Work out the finished part from the listing and answer in its coordinate system (mm). A direction names the side the tool comes from. Coordinates: 2 decimals unless noted, no trailing zeros. Write each loop counter-clockwise with the first axis right and the second up, starting at its lowest first coordinate (ties: lowest second). Pieces come first, ordered by that corner, then holes. Notation, with made-up numbers: (15, 26) - (69, 26) arc R7 cw to (69, 36) - close; hole circle Ø3 at (57, 62.25). An arc over 180 degrees is marked (long way). Answer as a JSON object with one key per item and string values. Group by question number.
Autodesk Inventor part; units mm, degrees
ref_plane "YZ Plane" through (0, 0, 0) normal (1, 0, 0) x (0, 1, 0)
ref_plane "XZ Plane" through (0, 0, 0) normal (0, 1, 0) x (-1, 0, 0)
ref_plane "XY Plane" through (0, 0, 0) normal (0, 0, 1) x (1, 0, 0)
sketch "Sketch1" plane through (0, 0, 0) normal (1, 0, 0) x (0, 1, 0)
  line L0 (-10, 10) -> (10, 10)
  line L1 (10, 10) -> (10, -10)
  line L2 (10, -10) -> (-10, -10)
  line L3 (-10, -10) -> (-10, 10)
  line L4 (-10, 10) -> (10, -10) construction
  line L5 (10, 10) -> (-10, -10) construction
  line L6 (7, -7) -> (7, 7)
  line L7 (7, 7) -> (-7, 7)
  line L8 (-7, 7) -> (-7, -7)
  line L9 (-7, -7) -> (7, -7)
  point P0 (0, 0)
  dimension "d0" = 20
  dimension "d1" = 20
  dimension "d2" = 3
extrude "Extrusion1" add sketch "Sketch1" along normal blind 414
sketch "Sketch2" plane through (0, 10, 10) normal (0, 1, 0) x (1, 0, 0)
  circle A0 centre (17, 10) radius 2.75
  line L0 (0, 0) -> (0, 20)
  line L1 (0, 0) -> (414, 0)
  circle A1 centre (397, 10) radius 2.75
  line L2 (414, 20) -> (414, 0)
  circle A2 centre (37, 10) radius 2.75
  circle A3 centre (57, 10) radius 2.75
  circle A4 centre (77, 10) radius 2.75
  circle A5 centre (97, 10) radius 2.75
  circle A6 centre (117, 10) radius 2.75
  circle A7 centre (137, 10) radius 2.75
  circle A8 centre (157, 10) radius 2.75
  circle A9 centre (177, 10) radius 2.75
  circle A10 centre (197, 10) radius 2.75
  circle A11 centre (217, 10) radius 2.75
  circle A12 centre (237, 10) radius 2.75
  circle A13 centre (257, 10) radius 2.75
  circle A14 centre (277, 10) radius 2.75
  circle A15 centre (297, 10) radius 2.75
  circle A16 centre (317, 10) radius 2.75
  circle A17 centre (337, 10) radius 2.75
  circle A18 centre (357, 10) radius 2.75
  circle A19 centre (377, 10) radius 2.75
  circle A20 centre (397, 10) radius 2.75
  point P0 (0, 10)
  dimension "d5" = 5.5
  dimension "d6" = 17
  dimension "d7" = 10
  dimension "d8" = 5.5
  dimension "d9" = 10
  dimension "d10" = 17
  dimension "d13" = 20
extrude "Extrusion2" cut sketch "Sketch2" against normal blind 20
sketch "Sketch3" plane through (0, -10, 10) normal (0, 0, 1) x (1, 0, 0)
  circle A0 centre (17, 10) radius 2.75
  line L0 (0, 0) -> (0, 20)
  line L1 (0, 0) -> (414, 0)
  circle A1 centre (397, 10) radius 2.75
  line L2 (414, 20) -> (414, 0)
  circle A2 centre (37, 10) radius 2.75
  circle A3 centre (57, 10) radius 2.75
  circle A4 centre (77, 10) radius 2.75
  circle A5 centre (97, 10) radius 2.75
  circle A6 centre (117, 10) radius 2.75
  circle A7 centre (137, 10) radius 2.75
  circle A8 centre (157, 10) radius 2.75
  circle A9 centre (177, 10) radius 2.75
  circle A10 centre (197, 10) radius 2.75
  circle A11 centre (217, 10) radius 2.75
  circle A12 centre (237, 10) radius 2.75
  circle A13 centre (257, 10) radius 2.75
  circle A14 centre (277, 10) radius 2.75
  circle A15 centre (297, 10) radius 2.75
  circle A16 centre (317, 10) radius 2.75
  circle A17 centre (337, 10) radius 2.75
  circle A18 centre (357, 10) radius 2.75
  circle A19 centre (377, 10) radius 2.75
  circle A20 centre (397, 10) radius 2.75
  point P0 (0, 10)
  dimension "d29" = 5.5
  dimension "d31" = 17
  dimension "d30" = 10
  dimension "d26" = 5.5
  dimension "d28" = 10
  dimension "d27" = 17
  dimension "d21" = 20
extrude "Extrusion3" cut sketch "Sketch3" against normal blind 20
properties part number "2020 Extrusion Base" material "Aluminum 6061"
Q1. A tool of negligible diameter and unlimited length cuts with its end or side. For faces 1 (the face through (0, -9, 0)), 2 (the face through (204, 0, -7)), from which of +Z, -Z, +X, -X, +Y, -Y can it reach the whole face along a straight path? Write none if from no direction.
Q2. Section A-A on x = 327.5 is taken. Determine the outline of the cut face in (y, z), plus the area to 3 significant figures.
Q3. Consider L1, parallel to Z at x = 37, y = -8.75; L2, parallel to Z at x = 353, y = -1.5. Determine where each line is inside the solid, lowest interval first. Write a range as from..to.
Q4. For a pull along Z with two mould halves and no side action, classify faces 3 (the face through (204, 0, -10)), 4 (the face through (204, -7, 0)), 5 (the face through (414, -9, 0)) as +Z half, -Z half, draft (parallel to the pull), parting line (faces both ways), or undercut.
Q5. Flat-ended cylindrical pins translate along their axes: pin 1 Ø4.5 at (x, z) = (237, 0) entering from +Y; pin 2 Ø9 at (x, z) = (217, 0) entering from +Y. Find the tip coordinate at first contact, or state that the pin passes through.
Numbers:
{
 "1": {"face 1": "+Z, -Z, -X, +Y, -Y", "face 2": "+X, -X"},
 "2": {"outline": "(-10, -10) - (10, -10) - (10, 10) - (-10, 10) - close; hole (-7, -7) - (7, -7) - (7, 7) - (-7, 7) - close", "area": "204 mm²"},
 "3": {"L1": "z = -10..-2.75, 2.75..10", "L2": "z = -10..-7, 7..10"},
 "4": {"face 3": "-Z half", "face 4": "undercut", "face 5": "draft"},
 "5": {"pin 1": "passes through", "pin 2": "stops at y = 10"}
}
